from build123d import *

# Parameters (mm, degrees)
SKETCH_W        = 150
SKETCH_H        = 200
PAD_DEPTH       = 20
SKETCH001_W     = 146
SKETCH001_H     = 196
POCKET_DEPTH    = 2
SKETCH002_W     = 142
SKETCH002_H     = 192
POCKET001_DEPTH = 18


with BuildPart() as part:
    # Sketch → Pad (new body)
    with BuildSketch(Plane.XY):
        Rectangle(SKETCH_W, SKETCH_H)
    extrude(amount=PAD_DEPTH)

    # Sketch001 → Pocket (cut)
    with BuildSketch(Plane.XY.offset(20)):
        Rectangle(SKETCH001_W, SKETCH001_H)
    extrude(amount=-POCKET_DEPTH, mode=Mode.SUBTRACT)

    # Sketch002 → Pocket001 (cut)
    with BuildSketch(Plane.XY.offset(20)):
        Rectangle(SKETCH002_W, SKETCH002_H)
    extrude(amount=-POCKET001_DEPTH, mode=Mode.SUBTRACT)


solid = part.part
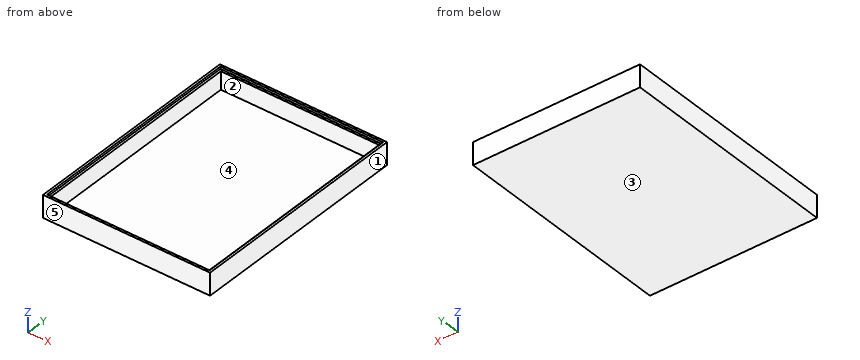
The model under review builds one solid part; all positions refer to its coordinate system, in mm. Face numbers are marked on the shaded views. A direction names the side the tool comes from. Coordinates: 2 decimals unless noted, no trailing zeros. Loops run counter-clockwise (first coordinate to the right, second up) from the corner with the lowest first, then second, coordinate; pieces in that order, holes last.
(1) Consider section A-A, the plane z = 11. Give the boundary of the cut face in (x, y), plus the area to 3 significant figures.
Determined:
outline: (-75, -100) - (75, -100) - (75, 100) - (-75, 100) - close; hole (-71, -96) - (71, -96) - (71, 96) - (-71, 96) - close
area: 2,740 mm2
(2) Wall thickness on L1, parallel to Y at x = -40.5, z = 3.25; L2, parallel to X at y = 25, z = 14.5; L3, parallel to X at y = 15.5, z = 18.5: over which ranges is each line inside the solid? List them lowest first.
Determined:
L1: y = -100 to -96, 96 to 100
L2: x = -75 to -71, 71 to 75
L3: x = -75 to -73, 73 to 75
(3) Consider section C-C, the plane x = -3. Give the boundary of the cut face in (y, z), plus the area to 3 significant figures.
Determined:
outline: (-100, 0) - (100, 0) - (100, 20) - (98, 20) - (98, 18) - (96, 18) - (96, 2) - (-96, 2) - (-96, 18) - (-98, 18) - (-98, 20) - (-100, 20) - close
area: 536 mm2
(4) Tool access review of the marked faces 1 and 2: name each direction out of +Z, -Z, +X, -X, +Y, -Y from which nothing blocks a thin tool from reaching the whole face with its end or side.
Determined:
face 1: +Z, -Z, +X, +Y, -Y
face 2: +Z
(5) Consider section B-B, the plane y = 83. Give the boundary of the cut face in (x, z), plus the area to 3 significant figures.
Determined:
outline: (-75, 0) - (75, 0) - (75, 20) - (73, 20) - (73, 18) - (71, 18) - (71, 2) - (-71, 2) - (-71, 18) - (-73, 18) - (-73, 20) - (-75, 20) - close
area: 436 mm2
(6) Draft analysis for pull direction Y (two halves, no side actions). For the marked faces 3, 4 and 5, state which applies: +Y half, -Y half, draft (parallel to the pull), parting line (faces both ways), or undercut.
Determined:
face 3: draft
face 4: undercut
face 5: -Y half
(7) Insertion check: P1, Ø2, axis at x = 1, y = 43, coming from the +Z side. The pin has a flat end and moves straight along its axis. Give the tip position at first contact, or say it passes through.
Determined:
P1: stops at z = 2
